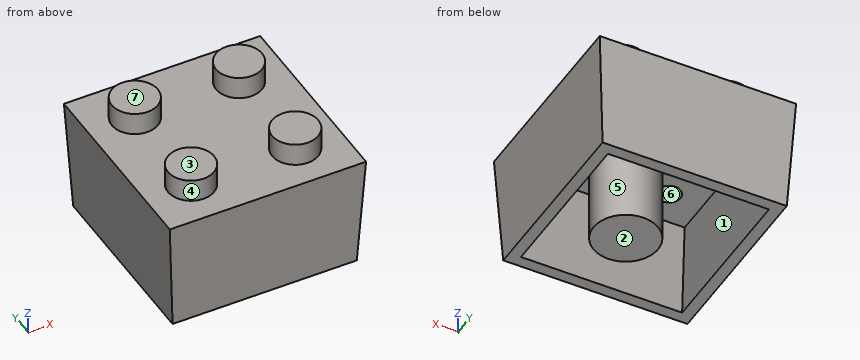
```python
from build123d import *

# Parameters (mm, degrees)
F0_W     = 16
F0_H     = 16
F1_DEPTH = 10
F1_TAPER = -3
F2_R     = 2
F3_DEPTH = 2
F4_T     = -1
F5_R     = 2.8
F6_DEPTH = 9


with BuildPart() as f1:
    # F0 (on Top) → F1 (new body)
    with BuildSketch(Plane.XY):
        Rectangle(F0_W, F0_H)
    extrude(amount=F1_DEPTH, taper=F1_TAPER)

    # F2 (on face) → F3 (join)
    with BuildSketch(Plane.XY.offset(10)):
        with Locations((-4.5240777928, 4.5240777928)):
            Circle(F2_R)
        with Locations((4.5240777928, 4.5240777928)):
            Circle(F2_R)
        with Locations((4.5240777928, -4.5240777928)):
            Circle(F2_R)
        with Locations((-4.5240777928, -4.5240777928)):
            Circle(F2_R)
    extrude(amount=F3_DEPTH)

    # F4
    f4_openings = [f1.faces().sort_by_distance(p)[0] for p in [
        (0, 0, 0),
    ]]
    offset(amount=F4_T, openings=f4_openings, kind=Kind.INTERSECTION)

    # F5 (on face) → F6 (join)
    with BuildSketch(Plane(origin=(0, 0, 9), x_dir=(1, 0, 0), z_dir=(0, 0, -1))):
        with Locations((1.0082904482, 1.2269222643)):
            Circle(F5_R)
    extrude(amount=F6_DEPTH)


solid = f1.part
```
Work out the finished part from the listing and answer in its coordinate system (mm). Face numbers are marked on the shaded views. A direction names the side the tool comes from. Round coordinates to 2 decimals unless told otherwise and drop trailing zeros. Write each loop counter-clockwise with the first axis right and the second up, starting at its lowest first coordinate (ties: lowest second). Pieces come first, ordered by that corner, then holes. Notation, with made-up numbers: (29.5, -23) - (61.5, -23) arc R13 cw to (61.5, -3) - close; hole circle Ø4 at (71.5, -27). An arc over 180 degrees is marked (long way). Return JSON: item names as keys, results as strings. Group by question number.
Q1. The mould has two halves that part along Y. Classify the marked faces 6 and 7: released by +Y, released by -Y, zero draft, split by the parting line, or undercut.
Q2. Find the intervals of material crossed by L1, parallel to Y at x = 0, z = 8; L2, parallel to X at y = -2.5, z = 2.5; L3, parallel to Y at x = 1.5, z = 8.25, in increasing order.
Q3. The part is cut by section A-A on z = 10.75. Write down the section's boundary in (x, y), then the cut area to 3 significant figures.
Q4. For the marked faces 1, 2, 3, 4 and 5, determine the directions among +Z, -Z, +X, -X, +Y, -Y from which every point of the face is accessible in a straight line to the end or side of a thin tool.
Q5. Each of these flat-tipped pins is pushed along its axis until it touches: pin 1 Ø2 at (x, y) = (-4.5, 4) entering from -Z; pin 2 Ø5 at (x, z) = (4.5, 5) entering from -Y; pin 3 Ø1.5 at (y, z) = (2.5, 1.5) entering from +X. Where does it stop, or does it pass through?
Q6. The part is cut by section B-B on z = 6. Count the separate pieces of the cut face and the enclosed holes in it, then the cut area to 3 significant figures.
Solved:
{
 "1": {"face 6": "undercut", "face 7": "zero draft"},
 "2": {"L1": "-8.42 to -7.42, -3.84 to 1.39, 7.42 to 8.42", "L2": "-8.13 to -7.13, -1.49 to 3.5, 7.13 to 8.13", "L3": "-8.43 to -7.43, -3.98 to 1.53, 7.43 to 8.43"},
 "3": {"outline": "circle Ø4 at (-4.52, -4.52); circle Ø4 at (-4.52, 4.52); circle Ø4 at (4.52, -4.52); circle Ø4 at (4.52, 4.52); hole circle Ø2 at (-4.52, -4.52); hole circle Ø2 at (-4.52, 4.52); hole circle Ø2 at (4.52, -4.52); hole circle Ø2 at (4.52, 4.52)", "area": "37.7 mm²"},
 "4": {"face 1": "none", "face 2": "-Z, +X, -X, +Y, -Y", "face 3": "+Z, +X, -X, +Y, -Y", "face 4": "+Z", "face 5": "-Z"},
 "5": {"pin 1": "z = 9", "pin 2": "y = -8.39", "pin 3": "x = 8.12"},
 "6": {"separate pieces": "2", "enclosed holes": "1", "area": "87.2 mm²"}
}
